Study the drawing (mm; zero at the part's minimum x, y, z) and answer. A direction names the side the tool comes from. Round coordinates to 2 decimals unless told otherwise and drop trailing zeros. Write each loop counter-clockwise with the first axis right and the second up, starting at its lowest first coordinate (ties: lowest second). Pieces come first, ordered by that corner, then holes.
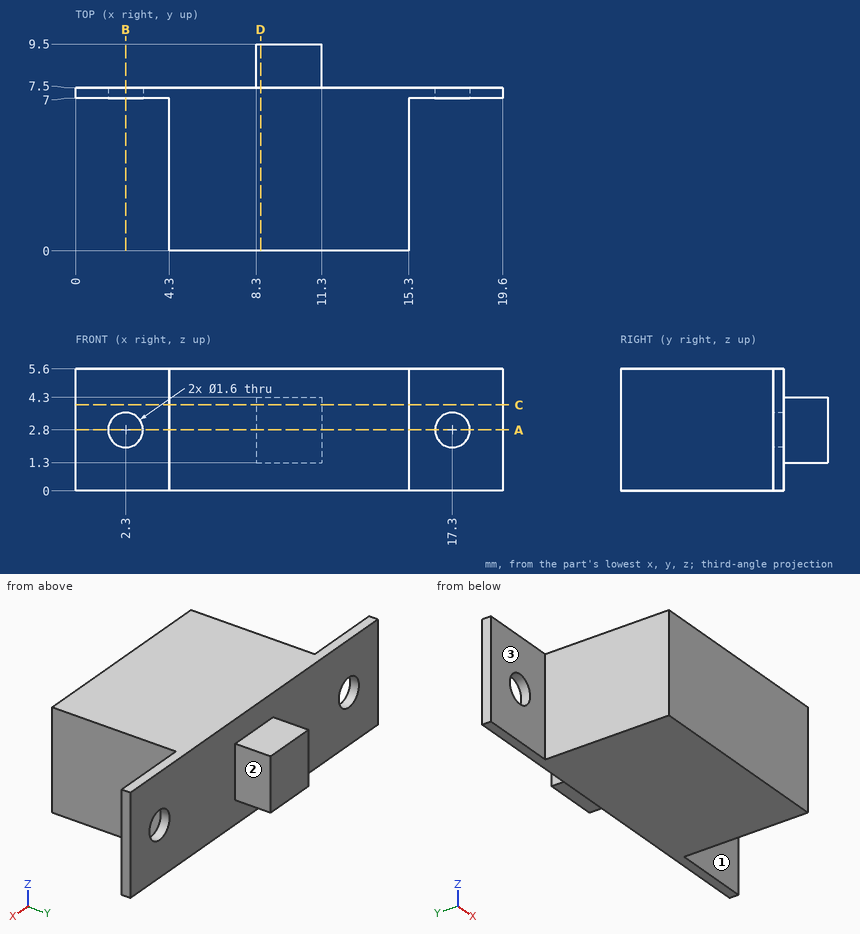
Q1. Find section C-C (z = 3.95). Determine the outline of the cut face in (x, y), plus the area to 3 significant figures.
Q2. Find the intervals of material crossed by L1, parallel to X at y = 7.3, z = 2.8; L2, parallel to Z at x = 2.3, y = 7.2; L3, parallel to Y at x = 16, z = 4.25, in increasing order.
Q3. Find section D-D (x = 8.5). Determine the outline of the cut face in (y, z), plus the area to 3 significant figures.
Q4. Find section A-A (z = 2.8). Determine the outline of the cut face in (x, y), plus the area to 3 significant figures.
Q5. Find section B-B (x = 2.3). Determine the outline of the cut face in (y, z).
Q6. Given pin 1 (2 mm diameter, centred on x = 16.5, z = 2.5, fed in from -Y); pin 2 (3 mm diameter, centred on y = 1, z = 4, fed in from +X); pin 3 (0.6 mm diameter, centred on y = 8.5, z = 3, fed in from -X), each flat-ended and moving along its own axis, determine where each tip first touches the part or whether it passes through.
Q7. A tool of negligible diameter and unlimited length cuts with its end or side. For the marked faces 1, 2 and 3, from which of +Z, -Z, +X, -X, +Y, -Y can it reach the whole face along a straight path? Write none if from no direction.
Report:
1. outline: (0, 7) - (4.3, 7) - (4.3, 0) - (15.3, 0) - (15.3, 7) - (19.6, 7) - (19.6, 7.5) - (11.3, 7.5) - (11.3, 9.5) - (8.3, 9.5) - (8.3, 7.5) - (0, 7.5) - close
1. area: 92.8 mm2
2. L1: x = 0 to 1.5, 3.1 to 16.5, 18.1 to 19.6
2. L2: z = 0 to 2, 3.6 to 5.6
2. L3: y = 7 to 7.5
3. outline: (0, 0) - (7.5, 0) - (7.5, 1.3) - (9.5, 1.3) - (9.5, 4.3) - (7.5, 4.3) - (7.5, 5.6) - (0, 5.6) - close
3. area: 48.0 mm2
4. outline: (0, 7) - (1.5, 7) - (1.5, 7.5) - (0, 7.5) - close; (3.1, 7) - (4.3, 7) - (4.3, 0) - (15.3, 0) - (15.3, 7) - (16.5, 7) - (16.5, 7.5) - (11.3, 7.5) - (11.3, 9.5) - (8.3, 9.5) - (8.3, 7.5) - (3.1, 7.5) - close; (18.1, 7) - (19.6, 7) - (19.6, 7.5) - (18.1, 7.5) - close
4. area: 91.2 mm2
5. outline: (7, 0) - (7.5, 0) - (7.5, 2) - (7, 2) - close; (7, 3.6) - (7.5, 3.6) - (7.5, 5.6) - (7, 5.6) - close
6. pin 1: stops at y = 7
6. pin 2: stops at x = 15.3
6. pin 3: stops at x = 8.3
7. face 1: +Z, -Z, +X, -Y
7. face 2: +Z, -Z, +X, +Y
7. face 3: +Z, -Z, -X, -Y
